Build history of the part. All positions in model axes, mm. Give positions to 0.01 mm unless a question says otherwise; leave off trailing zeros. Order: outer loops, then holes, each group sorted by start corner. A loop starts at its lowest first (then second) coordinate and runs counter-clockwise, first axis right, second up. Notation, with made-up numbers: M -6,78.5 L 31,78.5 A10 cw 31,94.5 Z; hole C -40,21 d7. An arc over 180 degrees is marked long. One line per item, written item: value.
from build123d import *

# Parameters (mm, degrees)
SKETCH1_R      = 3.4
EXTRUDE1_DEPTH = 1.85


# Read off the part's stored shape, not the designer's step: Cut-Extrude1
with BuildPart() as part:
    # Sketch1 → Extrude1 (new, symmetric)
    with BuildSketch(Plane(origin=(0, 0, 0), x_dir=(0, 0, -1), z_dir=(1, 0, 0))):
        Polygon((7.505553499, 0), (3.75277675, 6.5), (-3.75277675, 6.5), (-7.505553499, 0), (-3.75277675, -6.5), (3.75277675, -6.5), align=None)
        Circle(SKETCH1_R, mode=Mode.SUBTRACT)
    extrude(amount=EXTRUDE1_DEPTH, both=True)

    # Cut-Extrude1 outline → Cut-Extrude1 (revolve, cut)
    with BuildSketch(Plane.YX):
        Polygon((7.505553503, 1.850001347), (6.499998254, 1.850001347), (7.505553503, 1.269443414), align=None)
    cut_extrude1 = revolve(axis=Axis((0, 0, 0), (1, 0, 0)), mode=Mode.SUBTRACT)

    # Mirror1: Cut-Extrude1 across plane
    add(cut_extrude1.mirror(Plane(origin=(0, 0, 0), x_dir=(0, 0, 1), z_dir=(1, 0, 0))), mode=Mode.SUBTRACT)


solid = part.part
1) Saw through at B-B, the plane x = 1.6. Write the cut outline in (y, z).
Check values:
outline: M -6.5,-2.41 A6.93 ccw -5.34,-4.42 L -1.16,-6.84 A6.93 ccw 1.16,-6.84 L 5.34,-4.42 A6.93 ccw 6.5,-2.41 L 6.5,2.41 A6.93 ccw 5.34,4.42 L 1.16,6.84 A6.93 ccw -1.16,6.84 L -5.34,4.42 A6.93 ccw -6.5,2.41 Z; hole C 0,0 d6.8
2) Pin check, flat tips, straight feed: pin 1 (2 mm diameter, centred on x = 0, z = 6, fed in from -Y); pin 2 (1.5 mm diameter, centred on x = -1, y = -3.5, fed in from +Z). Stop position of each tip, or through.
Check values:
pin 1: y = -4.34
pin 2: z = 5.92
3) Drill centre lines: probe 1 along Y at (x, z) = (0.45, 0); probe 2 along Z at (x, y) = (1.3, 0.75); probe 3 along Y at (x, z) = (-0.1, -1.25). Where is each one in solid material? Low to high. Write a range as from..to.
Check values:
probe 1: -6.5..-3.4, 3.4..6.5
probe 2: -7.07..-3.32, 3.32..7.07
probe 3: -6.5..-3.16, 3.16..6.5
4) Mould opens along Y. For faces 1 (the face through (-0.03, -3.32, 0.74)), 2 (the face through (1.85, -3, -3)), 3 (the face through (1.71, -5.83, 3.39)), 4 (the face through (1.71, 5.83, -3.39)) say: released by +Y, released by -Y, zero draft, split by the parting line, or undercut.
Check values:
face 1: undercut
face 2: zero draft
face 3: released by -Y
face 4: released by +Y
5) Saw through at A-A, the plane x = -0.65. Write the cut outline in (y, z).
Check values:
outline: M -6.5,-3.75 L 0,-7.51 L 6.5,-3.75 L 6.5,3.75 L 0,7.51 L -6.5,3.75 Z; hole C 0,0 d6.8
